from build123d import *

# Parameters (mm, degrees)
SKETCH_1_R       = 1.585
EXTRUDE_1_DEPTH  = 1.6
SKETCH_2_W       = 5.1
SKETCH_2_H       = 86.4
EXTRUDE_2_DEPTH  = 8
SKETCH_3_W       = 16.4
SKETCH_3_H       = 22.2
EXTRUDE_3_DEPTH  = 13
SKETCH_4_W       = 14.42
SKETCH_4_H       = 13.5
EXTRUDE_4_DEPTH  = 6
SKETCH_5_W       = 24.3
SKETCH_5_H       = 6.4
EXTRUDE_5_DEPTH  = 2
SKETCH_6_W       = 10
SKETCH_6_H       = 12
EXTRUDE_6_DEPTH  = 2
SKETCH_7_W       = 15
SKETCH_7_H       = 15
EXTRUDE_7_DEPTH  = 2
SKETCH_8_W       = 13
SKETCH_8_H       = 10
EXTRUDE_8_DEPTH  = 6
SKETCH_9_W       = 9
SKETCH_9_H       = 7
EXTRUDE_9_DEPTH  = 3
SKETCH_10_W      = 10
SKETCH_10_H      = 12
EXTRUDE_10_DEPTH = 7
SKETCH_11_R      = 3.25
EXTRUDE_11_DEPTH = 6
SKETCH_12_W      = 14.7
SKETCH_12_H      = 4.6
SKETCH_12_W_2    = 5
SKETCH_12_H_2    = 23.9
EXTRUDE_12_DEPTH = 2
SKETCH_14_W      = 5
SKETCH_14_H      = 4
SKETCH_14_W_2    = 2
EXTRUDE_13_DEPTH = 2


with BuildPart() as part:
    # 草图1 → 凸台-拉伸1 (new body)
    with BuildSketch(Plane.XY):
        with BuildLine():
            Line((81.28, 82.72), (-13.36, 82.72))
            Line((-13.36, 82.72), (-13.36, 75.84))
            Line((-13.36, 75.84), (-5.19, 75.84))
            Line((-5.19, 75.84), (-5.19, 57.56))
            Line((-5.19, 57.56), (-13.36, 57.56))
            Line((-13.36, 57.56), (-13.36, 49.59))
            Line((-13.36, 49.59), (-6.94, 49.59))
            ThreePointArc((-6.94, 49.59), (-5.115, 47.765), (-6.94, 45.94))
            Line((-6.94, 45.94), (-17.88, 45.94))
            Line((-17.88, 45.94), (-17.88, 34.72))
            Line((-17.88, 34.72), (-10.42, 34.72))
            ThreePointArc((-10.42, 34.72), (-9.495, 33.795), (-10.42, 32.87))
            Line((-10.42, 32.87), (-17.88, 32.87))
            Line((-17.88, 32.87), (-17.88, 11.64))
            Line((-17.88, 11.64), (-5.11, 11.64))
            Line((-5.11, 11.64), (-5.11, -13.88))
            Line((-5.11, -13.88), (81.28, -13.88))
            Line((81.28, -13.88), (81.28, 82.72))
        make_face()
        with Locations((48.92, 64.16)):
            Circle(SKETCH_1_R, mode=Mode.SUBTRACT)
        with Locations((4.42, 64.16)):
            Circle(SKETCH_1_R, mode=Mode.SUBTRACT)
        with Locations((4.42, 4.42)):
            Circle(SKETCH_1_R, mode=Mode.SUBTRACT)
        with Locations((48.92, 4.42)):
            Circle(SKETCH_1_R, mode=Mode.SUBTRACT)
        with Locations((72.92, -9.58)):
            Circle(SKETCH_1_R, mode=Mode.SUBTRACT)
        with Locations((72.92, 78.42)):
            Circle(SKETCH_1_R, mode=Mode.SUBTRACT)
        with Locations((-9.76, 79.42)):
            Circle(SKETCH_1_R, mode=Mode.SUBTRACT)
        with Locations((-9.26, 53.56)):
            Circle(SKETCH_1_R, mode=Mode.SUBTRACT)
    extrude(amount=EXTRUDE_1_DEPTH)

    # 草图2 → 凸台-拉伸2 (add)
    with BuildSketch(Plane.XY.offset(1.6)):
        with Locations((78.73, 34.62)):
            Rectangle(SKETCH_2_W, SKETCH_2_H)
    extrude(amount=EXTRUDE_2_DEPTH)

    # 草图3 → 凸台-拉伸3 (add)
    with BuildSketch(Plane.XY.offset(1.6)):
        with Locations((61.38, 71.62)):
            Rectangle(SKETCH_3_W, SKETCH_3_H)
    extrude(amount=EXTRUDE_3_DEPTH)

    # 草图4 → 凸台-拉伸4 (add)
    with BuildSketch(Plane.XY.offset(1.6)):
        with Locations((41.97, 75.97)):
            Rectangle(SKETCH_4_W, SKETCH_4_H)
    extrude(amount=EXTRUDE_4_DEPTH)

    # 草图5 → 凸台-拉伸5 (add)
    with BuildSketch(Plane.XY.offset(1.6)):
        with Locations((19.13, 79.52)):
            Rectangle(SKETCH_5_W, SKETCH_5_H)
    extrude(amount=EXTRUDE_5_DEPTH)

    # 草图6 → 凸台-拉伸6 (add)
    with BuildSketch(Plane.XY.offset(1.6)):
        with Locations((1.64, 76.72)):
            Rectangle(SKETCH_6_W, SKETCH_6_H)
    extrude(amount=EXTRUDE_6_DEPTH)

    # 草图7 → 凸台-拉伸7 (add)
    with BuildSketch(Plane.XY.offset(1.6)):
        with Locations((60.78, -6.38)):
            Rectangle(SKETCH_7_W, SKETCH_7_H)
    extrude(amount=EXTRUDE_7_DEPTH)

    # 草图8 → 凸台-拉伸8 (add)
    with BuildSketch(Plane.XY.offset(1.6)):
        with Locations((42.28, -8.88)):
            Rectangle(SKETCH_8_W, SKETCH_8_H)
    extrude(amount=EXTRUDE_8_DEPTH)

    # 草图9 → 凸台-拉伸9 (add)
    with BuildSketch(Plane.XY.offset(1.6)):
        with Locations((26.78, -10.38)):
            Rectangle(SKETCH_9_W, SKETCH_9_H)
    extrude(amount=EXTRUDE_9_DEPTH)

    # 草图10 → 凸台-拉伸10 (add)
    with BuildSketch(Plane.XY.offset(1.6)):
        with Locations((1.89, -7.88)):
            Rectangle(SKETCH_10_W, SKETCH_10_H)
    extrude(amount=EXTRUDE_10_DEPTH)

    # 草图11 → 凸台-拉伸11 (add)
    with BuildSketch(Plane.XY.offset(1.6)):
        with Locations((10.89, -8.28)):
            Circle(SKETCH_11_R)
    extrude(amount=EXTRUDE_11_DEPTH)

    # 草图12 → 凸台-拉伸12 (add)
    with BuildSketch(Plane(origin=(0, 0, 0), x_dir=(-1, 0, 0), z_dir=(0, 0, -1))):
        with Locations((-61.83, 12.42)):
            Rectangle(SKETCH_12_W, SKETCH_12_H)
        with Locations((-9.78, 25.07)):
            Rectangle(SKETCH_12_W_2, SKETCH_12_H_2)
    extrude(amount=EXTRUDE_12_DEPTH)

    # 草图14 → 凸台-拉伸13 (add)
    with BuildSketch(Plane(origin=(0, 0, 0), x_dir=(-1, 0, 0), z_dir=(0, 0, -1))):
        with Locations((-10.39, -8.88)):
            Rectangle(SKETCH_14_W, SKETCH_14_H)
        with Locations((-20.89, -1.88)):
            Rectangle(SKETCH_14_W_2, SKETCH_14_H)
    extrude(amount=EXTRUDE_13_DEPTH)


solid = part.part
Could you check a few things on this model? Use its own coordinates, in mm. A direction names the side the tool comes from. Give positions to 0.01 mm unless a question says otherwise; leave off trailing zeros. Write each loop counter-clockwise with the first axis right and the second up, starting at its lowest first coordinate (ties: lowest second). Pieces come first, ordered by that corner, then holes. Notation, with made-up numbers: (-6, 87.5) -> (47, 87.5) arc R23 ccw to (47, 107.5) -> close; hole circle Ø1 at (12.5, -30.75). An arc over 180 degrees is marked (long way). Write each question's results on one line, items separated by ' | '. Start each with the question number.
Q1. Suppose I cut it at D-D, the plane y = 73.5. List the corners of the cut face in (x, z) for me, and give its area (3 significant figures).
Q2. We'd pull the mould along Y, two halves only. Please class faces 1 (the face through (13.892, -9.525, 4.558)), 2 (the face through (2, -8, 8.6)), 3 (the face through (79, -8.58, 6)): +Y half, -Y half, draft (parallel to the pull), parting line (faces both ways), or undercut.
Q3. Suppose I cut it at A-A, the plane y = 53.56. List the corners of the cut face in (x, z) for me (3 decimals).
Q4. I'm going to push flat-ended pins straight in: pin 1 Ø4 at (x, y) = (48.92, 64.16) entering from -Z; pin 2 Ø6.5 at (y, z) = (-10.5, 5.5) entering from -X; pin 3 Ø7 at (x, y) = (11, -8.5) entering from +Z. Where does each tip first touch, or does it pass through?
Q5. Suppose I cut it at C-C, the plane z = 6. List the corners of the cut face in (x, y) for me, and give its area (3 significant figures).
Q6. Which directions (+Z, -Z, +X, -X, +Y, -Y) give clear straight access to the entire face, cutting with the end or side of a thin tool? Please do faces 4 (the face through (49.18, 76, 5)), 5 (the face through (79, 77.82, 6)), 6 (the face through (42, 76, 7.6)), 7 (the face through (-3.11, -8, 5)), 8 (the face through (35.78, -9, 5)).
Q7. I need wall thicknesses on probe 1 along Y at (x, z) = (4.42, 0.6) (3 decimals); probe 2 along X at (y, z) = (64.16, 1.15) (3 decimals); probe 3 along Y at (x, z) = (72.92, 0.55) (3 decimals). Which ranges of each line are inside material? Lowest first, please.
Q8. Suppose I cut it at B-B, the plane x = 4.42. List the corners of the cut face in (y, z) for me (3 decimals).
Outcome:
1) outline: (-5.19, 0) -> (81.28, 0) -> (81.28, 9.6) -> (76.18, 9.6) -> (76.18, 1.6) -> (69.58, 1.6) -> (69.58, 14.6) -> (53.18, 14.6) -> (53.18, 1.6) -> (49.18, 1.6) -> (49.18, 7.6) -> (34.76, 7.6) -> (34.76, 1.6) -> (6.64, 1.6) -> (6.64, 3.6) -> (-3.36, 3.6) -> (-3.36, 1.6) -> (-5.19, 1.6) -> close | area: 499 mm2
2) face 1: undercut | face 2: draft | face 3: -Y half
3) outline: (-13.36, 0) -> (-10.845, 0) -> (-10.845, 1.6) -> (-13.36, 1.6) -> close; (-7.675, 0) -> (81.28, 0) -> (81.28, 9.6) -> (76.18, 9.6) -> (76.18, 1.6) -> (-7.675, 1.6) -> close
4) pin 1: z = 0 | pin 2: x = -3.11 | pin 3: z = 7.6
5) outline: (-3.11, -13.88) -> (6.89, -13.88) -> (6.89, -1.88) -> (-3.11, -1.88) -> close; circle Ø6.5 at (10.89, -8.28); (34.76, 69.22) -> (49.18, 69.22) -> (49.18, 82.72) -> (34.76, 82.72) -> close; (35.78, -13.88) -> (48.78, -13.88) -> (48.78, -3.88) -> (35.78, -3.88) -> close; (53.18, 60.52) -> (69.58, 60.52) -> (69.58, 82.72) -> (53.18, 82.72) -> close; (76.18, -8.58) -> (81.28, -8.58) -> (81.28, 77.82) -> (76.18, 77.82) -> close | area: 1,280 mm2
6) face 4: +Z, +Y, -Y | face 5: +Z, +X, +Y | face 6: +Z, -X, +Y, -Y | face 7: +Z, -X, -Y | face 8: +Z, -Y
7) probe 1: -13.88 to 2.835, 6.005 to 62.575, 65.745 to 82.72 | probe 2: -5.19 to 2.835, 6.005 to 47.335, 50.505 to 81.28 | probe 3: -13.88 to -11.165, -7.995 to 76.835, 80.005 to 82.72
8) outline: (-13.88, 0) -> (2.835, 0) -> (2.835, 1.6) -> (-1.88, 1.6) -> (-1.88, 8.6) -> (-13.88, 8.6) -> close; (6.005, 0) -> (62.575, 0) -> (62.575, 1.6) -> (6.005, 1.6) -> close; (65.745, 0) -> (82.72, 0) -> (82.72, 3.6) -> (70.72, 3.6) -> (70.72, 1.6) -> (65.745, 1.6) -> close
